Design review of the part built by this model. Coordinates are the model's own, in mm. A direction names the side the tool comes from. Coordinates: 2 decimals unless noted, no trailing zeros. Loops run counter-clockwise (first coordinate to the right, second up) from the corner with the lowest first, then second, coordinate; pieces in that order, holes last. Notation, with made-up numbers: M 45.5,49.25 L 89.5,49.25 A24 cw 89.5,70.25 Z; hole C 41.25,-14.75 d6. An arc over 180 degrees is marked long. One line per item, written item: value.
Autodesk Inventor part; units mm, degrees
ref_plane "YZ Plane" through (0, 0, 0) normal (1, 0, 0) x (0, 1, 0)
ref_plane "XZ Plane" through (0, 0, 0) normal (0, 1, 0) x (-1, 0, 0)
ref_plane "XY Plane" through (0, 0, 0) normal (0, 0, 1) x (1, 0, 0)
sketch "Sketch1" plane through (0, 0, 0) normal (0, 0, 1) x (1, 0, 0)
  circle A0 centre (0, 0) radius 5.15
  circle A1 centre (0, 0) radius 16
  line L0 (-16, 0) -> (-16, -20)
  line L1 (-16, -20) -> (16, -20)
  line L2 (16, -20) -> (16, 0)
  circle A2 centre (0, 0) radius 14.5
  point P0 (-8, 0)
  point P1 (8, 0)
  dimension "d0" = 10.3
  dimension "d1" = 32
  dimension "d3" = 20
  dimension "d4" = 8
  dimension "d5" = 8
  dimension "d28" = 1.5
extrude "Extrusion1" add sketch "Sketch1" along normal blind 3 contours A1 | L2 L1 L0 A1 | A2
hole "Hole1" at (-8, 0, 0) at (8, 0, 0) direction (0, 0, 1) diameter 2.3 end through all
sketch "Sketch2" plane through (0, 0, 0) normal (0, 0, -1) x (-1, 0, 0)
  arc A0 (1.3828, 14.685) -> (-1.3828, 14.685) centre (0, 0) ccw
  line L0 (-1.3828, 14.685) -> (-1.5, 15.9295)
  arc A1 (16, 0) -> (-16, 0) centre (0, 0) ccw
  line L1 (1.3828, 14.685) -> (1.5, 15.9295)
  point P0 (0, 14.75)
  dimension "d15" = 3
  dimension "d16" = 1.25
extrude "Extrusion2" add sketch "Sketch2" along normal blind 15
sketch "Sketch3" plane through (0, 0, 0) normal (0, 0, -1) x (-1, 0, 0)
  arc A0 (-1.9403, 14.7378) -> (1.9403, 14.7378) centre (0, 0) ccw
  arc A1 (-2.3319, 17.7122) -> (2.3319, 17.7122) centre (0, 0) ccw
  line L0 (-6, -16.8273) -> (-6, -20)
  line L1 (-6, -20) -> (6, -20)
  line L2 (16, -20) -> (-16, -20) construction
  line L3 (6, -16.8273) -> (6, -20)
  line L4 (-12, -13.2347) -> (-9.9849, -11.0123)
  line L5 (12, -13.2347) -> (9.9849, -11.0123)
  point P0 (0, 0)
  dimension "d19" = 3
  dimension "d20" = 12
  dimension "d21" = 24
  dimension "d22" = 12
extrude "Extrusion3" add sketch "Sketch3" along normal blind 40
chamfer "Chamfer1" distance 0.5 angle 45 2 edges at (-8, -1.15, 3) (8, -1.15, 3)
sketch "Sketch4" plane through (0, 0, -40) normal (0, 0, -1) x (-1, 0, 0)
  line L0 (-6, -20) -> (6, -20)
  line L1 (6, -20) -> (6, -16.8273)
  line L2 (6, -20) -> (6, -16)
  line L3 (6, -16) -> (-6, -16)
  line L4 (-6, -16.8273) -> (-6, -20)
  line L5 (-6, -16) -> (-6, -20)
  point P0 (0, 0)
  dimension "d29" = 4
extrude "Extrusion4" add sketch "Sketch4" along normal blind 18
sketch "Sketch6" plane through (0, 0, -58) normal (0, 0, -1) x (-1, 0, 0)
  line L0 (-4.65, -16.85) -> (4.65, -16.85)
  line L1 (4.65, -16.85) -> (4.65, -19.15)
  line L2 (4.65, -19.15) -> (-4.65, -19.15)
  line L3 (-4.65, -19.15) -> (-4.65, -16.85)
  line L4 (-6, -20) -> (6, -20)
  line L5 (6, -20) -> (6, -16)
  point P0 (0, 0)
  point P1 (0, -16.85)
  point P2 (0, -20)
  point P3 (4.65, -18)
  point P4 (6, -18)
  dimension "d36" = 2.3
  dimension "d37" = 9.3
extrude "Extrusion5" cut sketch "Sketch6" against normal blind 6
properties part number "Motor Face Mount Mk2"
(1) We need section D-D on x = 8. State the section outline as (y, z) points, then the cut area to 3 significant figures.
Reply:
outline: M -20,0 L -15.97,0 L -15.97,-40 L -12.53,-40 L -12.53,0 L -1.15,0 L -1.15,2.5 L -1.65,3 L -20,3 Z; M 1.15,0 L 13.86,0 L 13.86,3 L 1.65,3 L 1.15,2.5 Z
area: 232 mm2
(2) Insertion check: pin 1 (1.1 mm diameter, centred on x = -0.5, y = 15.5, fed in from -Z); pin 2 (8 mm diameter, centred on x = -6.5, y = 8.5, fed in from -Z); pin 3 (1.5 mm diameter, centred on x = 12, z = -13, fed in from +Y). Each pin has a flat end and moves straight along its axis. Give the tip position at first contact, or say it passes through.
Reply:
pin 1: stops at z = -15
pin 2: stops at z = 0
pin 3: stops at y = -12.41
(3) We need section B-B on y = -4. State the section outline as (x, z) points.
Reply:
outline: M -16,0 L -3.24,0 L -3.24,3 L -16,3 Z; M 3.24,0 L 16,0 L 16,3 L 3.24,3 Z
(4) We need section C-C on z = -10. State the section outline as (x, y) points (1 decimal), then the cut area to 3 significant figures.
Reply:
outline: M -12,-13.2 A17.9 ccw -6,-16.8 L -6,-20 L 6,-20 L 6,-16.8 A17.9 ccw 12,-13.2 L 10,-11 A14.9 cw -10,-11 Z; M -1.5,15.9 L -1.4,14.7 A14.7 cw 1.4,14.7 L 1.5,15.9 A16 ccw Z
area: 106 mm2
(5) We need section A-A on x = 0. State the section outline as (y, z) points, then the cut area to 3 significant figures.
Reply:
outline: M -20,-58 L -19.15,-58 L -19.15,-52 L -16.85,-52 L -16.85,-58 L -16,-58 L -16,-40 L -14.86,-40 L -14.86,0 L -5.15,0 L -5.15,3 L -20,3 Z; M 5.15,0 L 14.75,0 L 14.75,-15 L 16,-15 L 16,3 L 5.15,3 Z
area: 359 mm2
(6) To check wall thickness, follow line 1 along Y through (x, z) = (0, 1.2); line 2 along Y through (x, z) = (-8, 1.9); line 3 along Z through (x, y) = (-0.5, -5.5). State the ranges of each line that lie inside material, in increasing order. Write a range as [from, to].
Reply:
line 1: y = [-20, -5.15], [5.15, 16]
line 2: y = [-20, -1.15], [1.15, 13.86]
line 3: z = [0, 3]
(7) Tool access review of faces 4 (the flat face through (-6, -18, -29)), 5 (the flat face through (0, -18, -52)), 6 (the flat face through (-11.01, -12.14, -19.72)), 7 (the flat face through (0, 15, -15)): name each direction out of +Z, -Z, +X, -X, +Y, -Y from which nothing blocks a thin tool from reaching the whole face with its end or side.
Reply:
face 4: -Z, -X, -Y
face 5: -Z
face 6: -Z, -X, +Y
face 7: -Z, +X, -X, +Y
(8) Mouldability with a two-part tool opening along Y and no side actions: class faces 1 (the flat face through (0, -20, -20)), 2 (the flat face through (0, -6, 3)), 3 (the cylindrical face through (0.02, 14.75, -7.4)) as released by +Y, released by -Y, zero draft, split by the parting line, or undercut.
Reply:
face 1: released by -Y
face 2: zero draft
face 3: undercut
